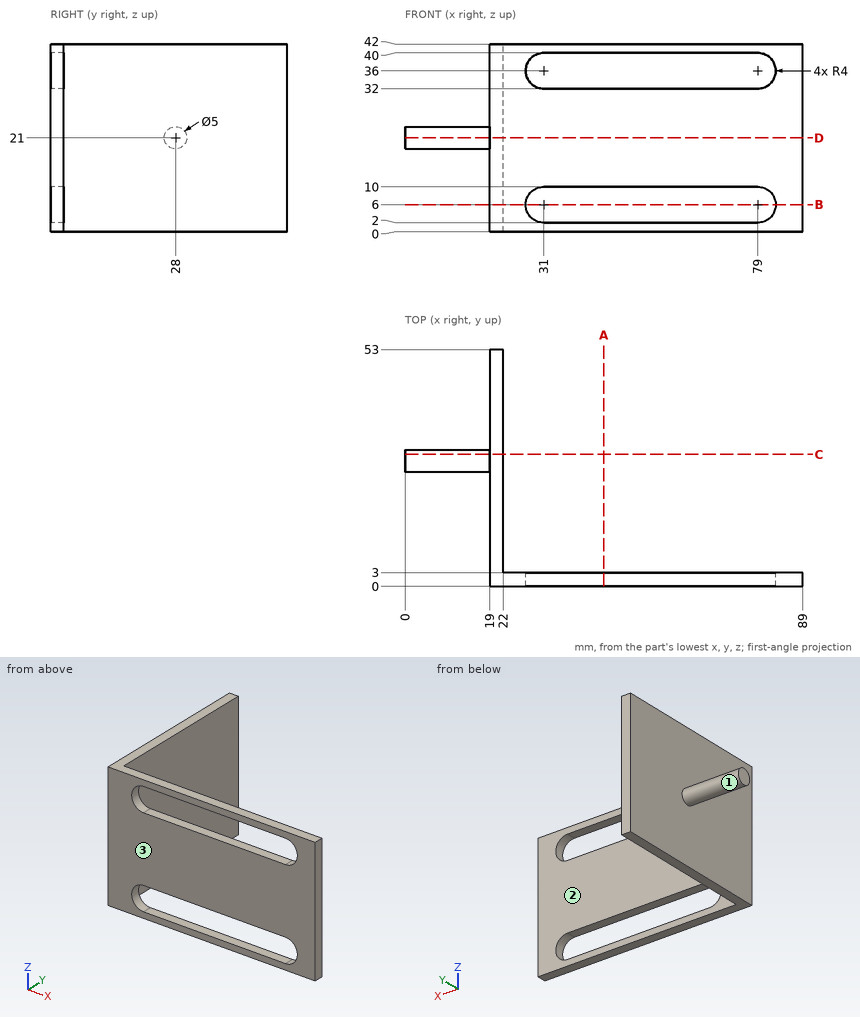
Input: dimensioned drawing with shaded views. Units: mm. Origin: part minimum x, y, z. A direction names the side the tool comes from. Give positions to 0.01 mm unless a question says otherwise; leave off trailing zeros. Loops run counter-clockwise (first coordinate to the right, second up) from the corner with the lowest first, then second, coordinate; pieces in that order, holes last. Notation, with made-up numbers: M 37,22.5 L 72,22.5 A17 ccw 72,40.5 Z; hole C 64.25,34 d2. An arc over 180 degrees is marked long. Put each result on its own line as item: value.
1) Reachability of the marked faces 1, 2 and 3 from +Z, -Z, +X, -X, +Y, -Y: full face, straight path, thin tool, end or side. Return the list, or none.
Computed values:
face 1: -X
face 2: +Z, -Z, +X, +Y
face 3: +Z, -Z, +X, -X, -Y
2) Material intervals for L1, parallel to Y at x = 72, z = 15.5; L2, parallel to X at y = 40.5, z = 30, sorted ascending. Write a range as from..to.
Computed values:
L1: y = 0..3
L2: x = 19..22
3) Cut plane D-D, the plane z = 21. Return the cut outline in (x, y), plus the area to 3 significant figures.
Computed values:
outline: M 0,25.5 L 19,25.5 L 19,0 L 89,0 L 89,3 L 22,3 L 22,53 L 19,53 L 19,30.5 L 0,30.5 Z
area: 455 mm^2
4) Cut plane A-A, the plane x = 44.5. Return the cut outline in (y, z).
Computed values:
outline: M 0,0 L 3,0 L 3,2 L 0,2 Z; M 0,10 L 3,10 L 3,32 L 0,32 Z; M 0,40 L 3,40 L 3,42 L 0,42 Z
5) Cut plane B-B, the plane z = 6. Return the cut outline in (x, y).
Computed values:
outline: M 19,0 L 27,0 L 27,3 L 22,3 L 22,53 L 19,53 Z; M 83,0 L 89,0 L 89,3 L 83,3 Z
6) Cut plane C-C, the plane y = 29.5. Return the cut outline in (x, z), plus the area to 3 significant figures.
Computed values:
outline: M 0,19 L 19,19 L 19,0 L 22,0 L 22,42 L 19,42 L 19,23 L 0,23 Z
area: 202 mm^2
7) First-contact query: P1, Ø8, axis at y = 44.5, z = 6.5, coming from the -X side; P2, Ø5, axis at y = 26.5, z = 17.5, coming from the +X side; P3, Ø10, axis at x = 28.5, z = 21, coming from the +Y side. Flat tips, straight axial feed; report the tip coordinate or a pass-through.
Computed values:
P1: stops at x = 19
P2: stops at x = 22
P3: stops at y = 3
